```python
from build123d import *

# Parameters (mm, degrees)
F0_R     = 63.5
F1_DEPTH = 12.7
F3_DEPTH = 25.4
F4_R     = 6.35
F5_R     = 19.05
F6_DEPTH = 38.101
F7_R     = 59.055
F7_R_2   = 45.085
F8_DEPTH = 6.35


with BuildPart() as f1:
    # F0 (on Front) → F1 (new body)
    with BuildSketch(Plane.XZ):
        Circle(F0_R)
    extrude(amount=F1_DEPTH)

    # F2 (on face) → F3 (join)
    with BuildSketch(Plane.XZ.offset(12.7)):
        with BuildLine():
            ThreePointArc((24.600173, -6.323884), (25.19925, -3.187132), (25.4, 0))
            ThreePointArc((25.4, 0), (25.19925, 3.187132), (24.600173, 6.323884))
            ThreePointArc((24.600173, 6.323884), (24.156836, 7.849032), (23.619044, 9.343489))
            ThreePointArc((23.619044, 9.343489), (20.549032, 14.929745), (16.184872, 19.575748))
            ThreePointArc((16.184872, 19.575748), (14.929745, 20.549032), (13.616243, 21.441967))
            ThreePointArc((13.616243, 21.441967), (7.849032, 24.156836), (1.5875, 25.350342))
            ThreePointArc((1.5875, 25.350342), (0, 25.4), (-1.5875, 25.350342))
            ThreePointArc((-1.5875, 25.350342), (-7.849032, 24.156836), (-13.616243, 21.441967))
            ThreePointArc((-13.616243, 21.441967), (-14.929745, 20.549032), (-16.184872, 19.575748))
            ThreePointArc((-16.184872, 19.575748), (-20.549032, 14.929745), (-23.619044, 9.343489))
            ThreePointArc((-23.619044, 9.343489), (-24.156836, 7.849032), (-24.600173, 6.323884))
            ThreePointArc((-24.600173, 6.323884), (-25.4, 0), (-24.600173, -6.323884))
            ThreePointArc((-24.600173, -6.323884), (-24.156836, -7.849032), (-23.619044, -9.343489))
            ThreePointArc((-23.619044, -9.343489), (-20.549032, -14.929745), (-16.184872, -19.575748))
            ThreePointArc((-16.184872, -19.575748), (-14.929745, -20.549032), (-13.616243, -21.441967))
            ThreePointArc((-13.616243, -21.441967), (-7.849032, -24.156836), (-1.5875, -25.350342))
            ThreePointArc((-1.5875, -25.350342), (0, -25.4), (1.5875, -25.350342))
            ThreePointArc((1.5875, -25.350342), (7.849032, -24.156836), (13.616243, -21.441967))
            ThreePointArc((13.616243, -21.441967), (14.929745, -20.549032), (16.184872, -19.575748))
            ThreePointArc((16.184872, -19.575748), (20.549032, -14.929745), (23.619044, -9.343489))
            ThreePointArc((23.619044, -9.343489), (24.156836, -7.849032), (24.600173, -6.323884))
        make_face()
        with BuildLine():
            ThreePointArc((23.619044, 9.343489), (24.156836, 7.849032), (24.600173, 6.323884))
            Line((24.600173, 6.323884), (54.796217, 16.135174))
            Line((54.796217, 16.135174), (54.305652, 17.644976))
            Line((54.305652, 17.644976), (53.815088, 19.154778))
            Line((53.815088, 19.154778), (23.619044, 9.343489))
        make_face()
        with BuildLine():
            Line((54.796217, -16.135174), (24.600173, -6.323884))
            ThreePointArc((24.600173, -6.323884), (24.156836, -7.849032), (23.619044, -9.343489))
            Line((23.619044, -9.343489), (53.815088, -19.154778))
            Line((53.815088, -19.154778), (54.305652, -17.644976))
            Line((54.305652, -17.644976), (54.796217, -16.135174))
        make_face()
        with BuildLine():
            ThreePointArc((13.616243, 21.441967), (14.929745, 20.549032), (16.184872, 19.575748))
            Line((16.184872, 19.575748), (34.847053, 45.262038))
            Line((34.847053, 45.262038), (33.562739, 46.195147))
            Line((33.562739, 46.195147), (32.278424, 47.128256))
            Line((32.278424, 47.128256), (13.616243, 21.441967))
        make_face()
        with BuildLine():
            Line((34.847053, -45.262038), (16.184872, -19.575748))
            ThreePointArc((16.184872, -19.575748), (14.929745, -20.549032), (13.616243, -21.441967))
            Line((13.616243, -21.441967), (32.278424, -47.128256))
            Line((32.278424, -47.128256), (33.562739, -46.195147))
            Line((33.562739, -46.195147), (34.847053, -45.262038))
        make_face()
        with BuildLine():
            ThreePointArc((-1.5875, 25.350342), (0, 25.4), (1.5875, 25.350342))
            Line((1.5875, 25.350342), (1.5875, 57.100342))
            Line((1.5875, 57.100342), (0, 57.100342))
            Line((0, 57.100342), (-1.5875, 57.100342))
            Line((-1.5875, 57.100342), (-1.5875, 25.350342))
        make_face()
        with BuildLine():
            Line((1.5875, -57.100342), (1.5875, -25.350342))
            ThreePointArc((1.5875, -25.350342), (0, -25.4), (-1.5875, -25.350342))
            Line((-1.5875, -25.350342), (-1.5875, -57.100342))
            Line((-1.5875, -57.100342), (0, -57.100342))
            Line((0, -57.100342), (1.5875, -57.100342))
        make_face()
        with BuildLine():
            ThreePointArc((-16.184872, 19.575748), (-14.929745, 20.549032), (-13.616243, 21.441967))
            Line((-13.616243, 21.441967), (-32.278424, 47.128256))
            Line((-32.278424, 47.128256), (-33.562739, 46.195147))
            Line((-33.562739, 46.195147), (-34.847053, 45.262038))
            Line((-34.847053, 45.262038), (-16.184872, 19.575748))
        make_face()
        with BuildLine():
            Line((-32.278424, -47.128256), (-13.616243, -21.441967))
            ThreePointArc((-13.616243, -21.441967), (-14.929745, -20.549032), (-16.184872, -19.575748))
            Line((-16.184872, -19.575748), (-34.847053, -45.262038))
            Line((-34.847053, -45.262038), (-33.562739, -46.195147))
            Line((-33.562739, -46.195147), (-32.278424, -47.128256))
        make_face()
        with BuildLine():
            ThreePointArc((-24.600173, 6.323884), (-24.156836, 7.849032), (-23.619044, 9.343489))
            Line((-23.619044, 9.343489), (-53.815088, 19.154778))
            Line((-53.815088, 19.154778), (-54.305652, 17.644976))
            Line((-54.305652, 17.644976), (-54.796217, 16.135174))
            Line((-54.796217, 16.135174), (-24.600173, 6.323884))
        make_face()
        with BuildLine():
            Line((-53.815088, -19.154778), (-23.619044, -9.343489))
            ThreePointArc((-23.619044, -9.343489), (-24.156836, -7.849032), (-24.600173, -6.323884))
            Line((-24.600173, -6.323884), (-54.796217, -16.135174))
            Line((-54.796217, -16.135174), (-54.305652, -17.644976))
            Line((-54.305652, -17.644976), (-53.815088, -19.154778))
        make_face()
    extrude(amount=F3_DEPTH)

    # F4
    f4_edges = [f1.edges().sort_by_distance(p)[0] for p in [
        (-16.184872, -25.4, 19.575748),
        (-1.5875, -25.4, 25.350342),
        (-24.600173, -25.4, 6.323884),
        (-24.600173, -25.4, -6.323884),
        (-23.619044, -25.4, -9.343489),
        (-16.184872, -25.4, -19.575748),
        (-13.616243, -25.4, -21.441967),
        (-1.5875, -25.4, -25.350342),
        (13.616243, -25.4, -21.441967),
        (1.5875, -25.4, -25.350342),
        (16.184872, -25.4, -19.575748),
        (23.619044, -25.4, -9.343489),
        (24.600173, -25.4, -6.323884),
        (24.600173, -25.4, 6.323884),
        (23.619044, -25.4, 9.343489),
        (16.184872, -25.4, 19.575748),
        (13.616243, -25.4, 21.441967),
        (1.5875, -25.4, 25.350342),
        (-13.616243, -25.4, 21.441967),
        (-23.619044, -25.4, 9.343489),
    ]]
    fillet(f4_edges, radius=F4_R)

    # F5 (on face) → F6 (cut, through all)
    with BuildSketch(Plane.XZ.offset(38.1)):
        Circle(F5_R)
    extrude(amount=-F6_DEPTH, mode=Mode.SUBTRACT)

    # F7 (on face) → F8 (cut)
    with BuildSketch(Plane(origin=(0, 0, 0), x_dir=(-1, 0, 0), z_dir=(0, 1, 0))):
        Circle(F7_R)
        Circle(F7_R_2, mode=Mode.SUBTRACT)
    extrude(amount=-F8_DEPTH, mode=Mode.SUBTRACT)


solid = f1.part
```
Geometry check sheet. Reference: the model listing, model coordinates, mm. A direction names the side the tool comes from. Coordinates: 2 decimals unless noted, no trailing zeros. Write each loop counter-clockwise with the first axis right and the second up, starting at its lowest first coordinate (ties: lowest second). Pieces come first, ordered by that corner, then holes. Notation, with made-up numbers: M 20.5,87 L 72.5,87 A16 ccw 72.5,106 Z; hole C 59.25,41 d4. An arc over 180 degrees is marked long. One line per item, written item: value. Start each with the question number.
(1) Depth check by flat-ended pin: pin 1 (7.5 mm diameter, centred on y = -20.5, z = -43, fed in from +X); pin 2 (1.6 mm diameter, centred on x = 0.5, y = -31.5, fed in from -Z); pin 3 (10 mm diameter, centred on y = -32.5, z = -14, fed in from +X); pin 4 (5 mm diameter, centred on x = 9.5, z = 28.5, fed in from +Y). Enter the tip coordinate at first touch or a pass-through.
(2) Sectioned sample at B-B, the plane y = -8.5. Enter the section's corners in (x, z), and give its area (3 significant figures).
(3) Scan lines: line 1 along Z through (x, y) = (0, -5) (3 decimals); line 2 along X through (y, z) = (-17.5, 25.5); line 3 along Z through (x, y) = (0, -10). Record each from-to range of solid material in increasing order. Write a range as [from, to].
(4) Sectioned sample at D-D, the plane z = 35. Enter the section's corners in (x, y), and give its area (3 significant figures).
(5) Tool access check on faces 5 (the face through (9.774, -3.131, -44.013)), 6 (the face through (-2.88, -25.58, 26.9)), 7 (the face through (41.46, -25.22, 15.14)). Record the directions out of +Z, -Z, +X, -X, +Y, -Y that give a thin tool (end or side, any length) a straight path to the whole face; none if there is none.
(6) Release check for a two-part mould opening along Z. For faces 1 (the face through (-24.423, -25.222, 36.317)), 2 (the face through (-18.143, -25.578, 20.069)), 3 (the face through (2.88, -25.58, -26.9)), 4 (the face through (-25.4, -25.2, 0)) record: released by +Z, released by -Z, zero draft, split by the parting line, or undercut.
(7) Sectioned sample at A-A, the plane x = 0. Enter the section's corners in (y, z) (3 decimals), and give its area (3 significant figures).
(8) Sectioned sample at C-C, the plane x = -51.5. Enter the section's corners in (y, z).
Filled sheet:
1. pin 1: x = 34.85
1. pin 2: z = -57.1
1. pin 3: x = 54.8
1. pin 4: y = 0
2. outline: C 0,0 d127; hole C 0,0 d38.1
2. area: 11,500 mm²
3. line 1: [-63.5, -59.055], [-45.085, -19.05], [19.05, 45.085], [59.055, 63.5]
3. line 2: [-20.49, -16.55], [-4.35, 4.35], [16.55, 20.49]
3. line 3: [-63.5, -19.05], [19.05, 63.5]
4. outline: M -52.98,-12.7 L -27.39,-12.7 L -27.39,-38.1 L -23.47,-38.1 L -23.47,-12.7 L -1.59,-12.7 L -1.59,-38.1 L 1.59,-38.1 L 1.59,-12.7 L 23.47,-12.7 L 23.47,-38.1 L 27.39,-38.1 L 27.39,-12.7 L 52.98,-12.7 L 52.98,0 L 47.57,0 L 47.57,-6.35 L 28.42,-6.35 L 28.42,0 L -28.42,0 L -28.42,-6.35 L -47.57,-6.35 L -47.57,0 L -52.98,0 Z
4. area: 1,380 mm²
5. face 5: +Y
5. face 6: +Z, -Y
5. face 7: -Y
6. face 1: released by +Z
6. face 2: undercut
6. face 3: released by -Z
6. face 4: undercut
7. outline: M -38.1,-57.1 L -12.7,-57.1 L -12.7,-63.5 L 0,-63.5 L 0,-59.055 L -6.35,-59.055 L -6.35,-45.085 L 0,-45.085 L 0,-19.05 L -38.1,-19.05 Z; M -38.1,19.05 L 0,19.05 L 0,45.085 L -6.35,45.085 L -6.35,59.055 L 0,59.055 L 0,63.5 L -12.7,63.5 L -12.7,57.1 L -38.1,57.1 Z
7. area: 2,880 mm²
8. outline: M -38.1,-18.4 L -12.7,-18.4 L -12.7,-37.15 L 0,-37.15 L 0,-28.9 L -6.35,-28.9 L -6.35,28.9 L 0,28.9 L 0,37.15 L -12.7,37.15 L -12.7,18.4 L -38.1,18.4 L -38.1,15.06 L -12.7,15.06 L -12.7,-15.06 L -38.1,-15.06 Z
